Check sheet for the modelled part. Datum: model origin and axes. Units: mm. Face numbers are marked on the shaded views. A direction names the side the tool comes from. Give positions to 0.01 mm unless a question says otherwise; leave off trailing zeros. Loops run counter-clockwise (first coordinate to the right, second up) from the corner with the lowest first, then second, coordinate; pieces in that order, holes last. Notation, with made-up numbers: (86, -21.5) -> (120, -21.5) arc R8 cw to (120, -16.5) -> close; hole circle Ø4 at (83.25, -36.5). An arc over 180 degrees is marked (long way). Answer as CSV lines item,"result". Start each with the question number.
(1) Section check C-C on x = -11. Enter the section's corners in (y, z) (3 decimals).
(2) Section check B-B on z = 20. Enter the section's corners in (x, y) (1 decimal).
(3) Material ranges on line 1 (Z direction, x = 1, y = -2) (3 decimals); line 2 (Z direction, x = -2.5, y = -9.5) (3 decimals); line 3 (Y direction, x = 10, z = 12) (3 decimals), recorded low to high. Write a range as from..to.
(4) Access from +Z, -Z, +X, -X, +Y, -Y to the whole of each face (thin tool, end or side, straight path). Record for the marked faces 1, 2 and 3.
(5) Gauge pin test, flat ends, axial feed: pin 1 Ø0.8 at (y, z) = (-0.5, 37) entering from +X (3 decimals); pin 2 Ø2.5 at (x, z) = (-10.64, 22.22) entering from -Y (3 decimals); pin 3 Ø2.5 at (x, z) = (10.64, 9.52) entering from +Y. Record the tip position at first contact, or that the pin passes through.
(6) Section check A-A on x = 0. Enter the section's corners in (y, z) (3 decimals), plus the area to 3 significant figures.
(7) Section check D-D on y = -2. State how many separate pieces and enclosed holes the cut face has, plus the area to 3 significant figures.
from build123d import *

# Parameters (mm, degrees)
F0_R     = 15.875
F1_DEPTH = 3.175
F2_W     = 26.67
F2_H     = 3.175
F3_DEPTH = 50.8
F4_W     = 9.525
F4_H     = 38.1
F5_DEPTH = 3.175
F6_W     = 15.875
F6_H     = 44.45
F7_DEPTH = 1
F8_R     = 1.016
F9_DEPTH = 3.175


with BuildPart() as f1:
    # F0 (on Top) → F1 (new body)
    with BuildSketch(Plane.XY):
        Circle(F0_R)
    extrude(amount=F1_DEPTH)

    # F2 (on face) → F3 (join)
    with BuildSketch(Plane.XY.offset(3.175)):
        with Locations((0, -1.5875)):
            Rectangle(F2_W, F2_H)
    extrude(amount=F3_DEPTH)

    # F4 (on face) → F5 (cut, through all)
    with BuildSketch(Plane(origin=(0, 0, 0), x_dir=(-1, 0, 0), z_dir=(0, 1, 0))):
        with Locations((0, 28.575)):
            Rectangle(F4_W, F4_H)
    extrude(amount=-F5_DEPTH, mode=Mode.SUBTRACT)

    # F6 (on face) → F7 (cut)
    with BuildSketch(Plane(origin=(0, 0, 0), x_dir=(-1, 0, 0), z_dir=(0, 1, 0))):
        with Locations((0, 28.575)):
            Rectangle(F6_W, F6_H)
    extrude(amount=-F7_DEPTH, mode=Mode.SUBTRACT)

    # F8 (on face) → F9 (cut, through all)
    with BuildSketch(Plane(origin=(0, 0, 0), x_dir=(-1, 0, 0), z_dir=(0, 1, 0))):
        with BuildLine():
            Line((10.63625, 9.525), (11.65225, 9.525))
            ThreePointArc((11.65225, 9.525), (10.63625, 10.541), (9.62025, 9.525))
            Line((9.62025, 9.525), (10.63625, 9.525))
        make_face()
        with BuildLine():
            ThreePointArc((9.62025, 9.525), (10.63625, 8.509), (11.65225, 9.525))
            Line((11.65225, 9.525), (10.63625, 9.525))
            Line((10.63625, 9.525), (9.62025, 9.525))
        make_face()
        with Locations((10.63625, 22.225)):
            Circle(F8_R)
        with Locations((10.63625, 34.925)):
            Circle(F8_R)
        with Locations((10.63625, 47.625)):
            Circle(F8_R)
        with Locations((-10.63625, 47.625)):
            Circle(F8_R)
        with Locations((-10.63625, 34.925)):
            Circle(F8_R)
        with Locations((-10.63625, 22.225)):
            Circle(F8_R)
        with Locations((-10.63625, 9.525)):
            Circle(F8_R)
    extrude(amount=-F9_DEPTH, mode=Mode.SUBTRACT)


solid = f1.part
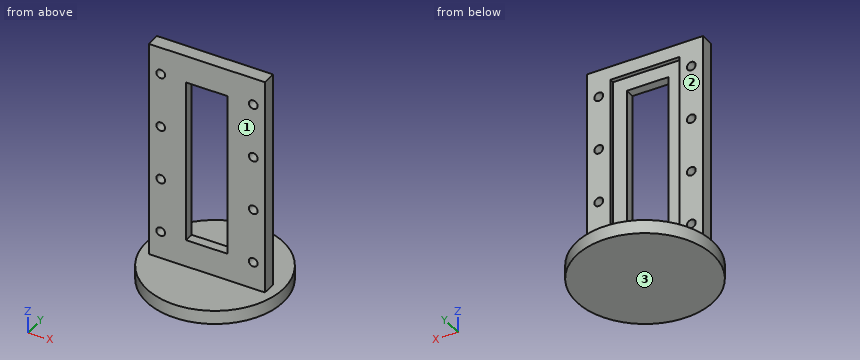
Working result:
1,outline,"(-11.446, 0) -> (11.446, 0) -> (11.446, 3.175) -> (0, 3.175) -> (0, 8.576) -> (-3.175, 8.576) -> (-3.175, 3.175) -> (-11.446, 3.175) -> close; (-3.175, 10.474) -> (0, 10.474) -> (0, 21.276) -> (-3.175, 21.276) -> close; (-3.175, 23.174) -> (0, 23.174) -> (0, 33.976) -> (-3.175, 33.976) -> close; (-3.175, 35.874) -> (0, 35.874) -> (0, 46.676) -> (-3.175, 46.676) -> close; (-3.175, 48.574) -> (0, 48.574) -> (0, 53.975) -> (-3.175, 53.975) -> close"
2,outline,"(-13.3, -3.2) -> (-4.8, -3.2) -> (-4.8, -1) -> (-7.9, -1) -> (-7.9, 0) -> (-13.3, 0) -> close; (4.8, -3.2) -> (13.3, -3.2) -> (13.3, 0) -> (7.9, 0) -> (7.9, -1) -> (4.8, -1) -> close"
3,line 1,"z = 0..9.525, 47.625..53.975"
3,line 2,"z = 0..3.175"
3,line 3,"y = -3.175..0"
4,face 1,"+Z, +X, -X, -Y"
4,face 2,"+Z, +X, -X, +Y"
4,face 3,"-Z, +X, -X, +Y, -Y"
5,pin 1,"stops at x = 13.335"
5,pin 2,"stops at y = -3.175"
5,pin 3,"stops at y = 0"
6,outline,"(-15.875, 0) -> (15.875, 0) -> (15.875, 3.175) -> (0, 3.175) -> (0, 6.35) -> (-1, 6.35) -> (-1, 9.525) -> (-3.175, 9.525) -> (-3.175, 3.175) -> (-15.875, 3.175) -> close; (-3.175, 47.625) -> (-1, 47.625) -> (-1, 50.8) -> (0, 50.8) -> (0, 53.975) -> (-3.175, 53.975) -> close"
6,area,"135 mm^2"
7,separate pieces,"1"
7,enclosed holes,"9"
7,area,"1,070 mm^2"
